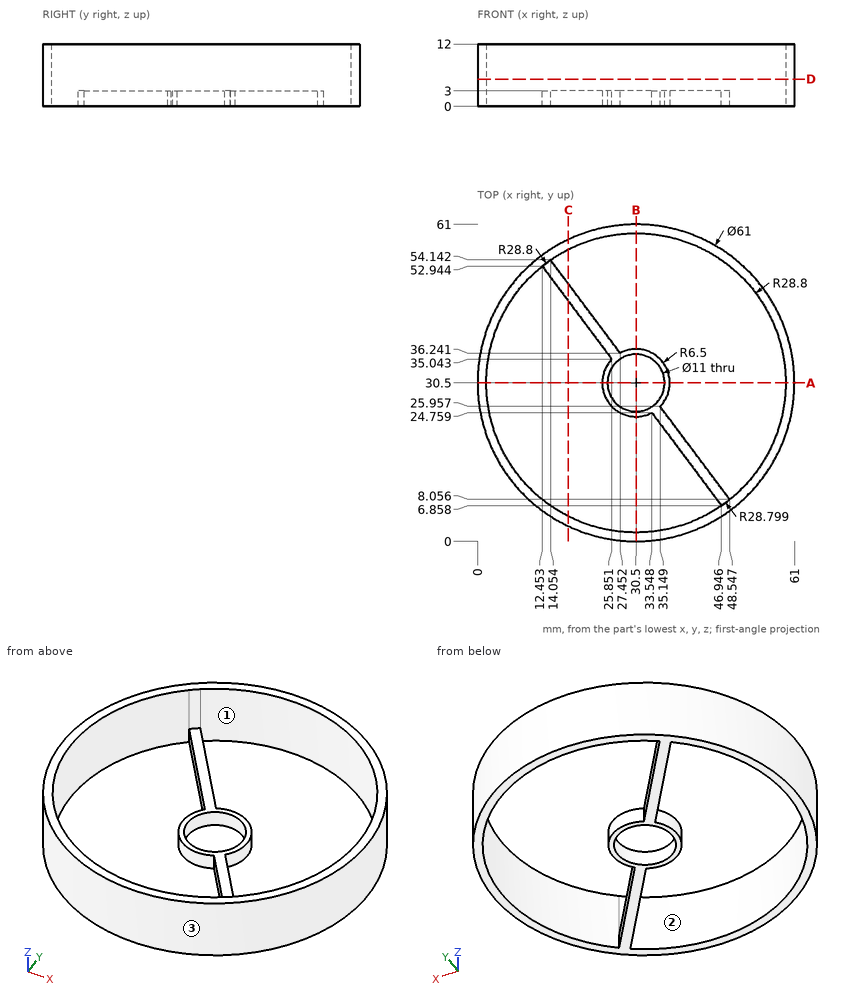
Verification items for this drawing (mm, ordinates from the low corner). Coordinates: 2 decimals unless noted, no trailing zeros. Order: outer loops, then holes, each group sorted by start corner. A loop starts at its lowest first (then second) coordinate and runs counter-clockwise, first axis right, second up. Notation, with made-up numbers: (10.25, 67.5) - (36.25, 67.5) arc R26 cw to (36.25, 101.5) - close; hole circle Ø10 at (56.5, 87). An arc over 180 degrees is marked (long way). Answer as a JSON object with one key per item and string values. Group by question number.
Item 1: Sectioned sample at A-A, the plane y = 30.5. Record the cut outline in (x, z).
Item 2: Sectioned sample at C-C, the plane x = 17.5. Record the cut outline in (y, z).
Item 3: Draft check along X on the marked faces 1, 2 and 3. Enter one of: +X half, -X half, draft (parallel to the pull), parting line (faces both ways), or undercut.
Item 4: Depth check by flat-ended pin: pin 1 Ø4 at (y, z) = (22.5, 2.5) entering from +X; pin 2 Ø1 at (y, z) = (46, 2.5) entering from +X; pin 3 Ø5 at (x, z) = (51, 2.5) entering from -Y. Enter the tip coordinate at first touch or a pass-through.
Item 5: Sectioned sample at D-D, the plane z = 5.25. Record the cut outline in (x, y).
Item 6: Scan lines: probe 1 along Y at (x, z) = (30.5, 1.75); probe 2 along X at (y, z) = (51.5, 2.25) (1 decimal); probe 3 along X at (y, z) = (24, 7.5). Record each from-to range of solid material in increasing order.
Resolved:
{
 "1": {"outline": "(0, 0) - (1.7, 0) - (1.7, 12) - (0, 12) - close; (24, 0) - (25, 0) - (25, 3) - (24, 3) - close; (36, 0) - (37, 0) - (37, 3) - (36, 3) - close; (59.3, 0) - (61, 0) - (61, 12) - (59.3, 12) - close"},
 "2": {"outline": "(2.91, 0) - (4.8, 0) - (4.8, 12) - (2.91, 12) - close; (46.2, 0) - (49.54, 0) - (49.54, 3) - (46.2, 3) - close; (56.2, 0) - (58.09, 0) - (58.09, 12) - (56.2, 12) - close"},
 "3": {"face 1": "undercut", "face 2": "undercut", "face 3": "parting line"},
 "4": {"pin 1": "x = 60.4", "pin 2": "x = 57.06", "pin 3": "y = 5.88"},
 "5": {"outline": "circle Ø61 at (30.5, 30.5); hole (12.45, 52.94) arc R28.8 ccw to (46.95, 6.86) arc R28.8 ccw to (48.55, 8.06) arc R28.8 ccw to (14.05, 54.14) arc R28.8 ccw to start"},
 "6": {"probe 1": "0 to 1.7, 24 to 25, 36 to 37, 59.3 to 61", "probe 2": "8.4 to 10.8, 13.5 to 16, 50.2 to 52.6", "probe 3": "0.7 to 2.44, 58.56 to 60.3"}
}
